Could you check a few things on this model? Use its own coordinates, in mm. A direction names the side the tool comes from. Round coordinates to 2 decimals unless told otherwise and drop trailing zeros. Loops run counter-clockwise (first coordinate to the right, second up) from the corner with the lowest first, then second, coordinate; pieces in that order, holes last. Notation, with made-up numbers: (82, 0.25) - (88, 0.25) arc R31 cw to (88, 39.25) - close; hole circle Ø4 at (89.25, 26). An arc over 180 degrees is marked (long way). Use one line per item in the form item = value.
```python
from build123d import *

# Parameters (mm, degrees)
F0_R          = 1.75
F1_DEPTH      = 1.65
F2_R          = 1
F3_W          = 15.5
F3_H          = 2.5
F4_DEPTH      = 2.25
F5_W          = 0.7
F5_H          = 0.7
F6_DEPTH      = 6
F6_DEPTH_BACK = 6
F7_R          = 0.75


with BuildPart() as f1:
    # F0 (on Top) → F1 (new body)
    with BuildSketch(Plane.XY):
        with BuildLine():
            Line((14.55, 6.8), (-14.55, 6.8))
            Line((-14.55, 6.8), (-14.55, 3.75))
            Line((-14.55, 3.75), (-14.55, 1.8708286934))
            ThreePointArc((-14.55, 1.8708286934), (-14.1771558135, 0.9682458366), (-14.05, 0))
            ThreePointArc((-14.05, 0), (-14.1771558135, -0.9682458366), (-14.55, -1.8708286934))
            Line((-14.55, -1.8708286934), (-14.55, -3.75))
            Line((-14.55, -3.75), (-14.55, -6.8))
            Line((-14.55, -6.8), (14.55, -6.8))
            Line((14.55, -6.8), (14.55, -3.75))
            Line((14.55, -3.75), (14.55, -1.8708286934))
            ThreePointArc((14.55, -1.8708286934), (14.05, 0), (14.55, 1.8708286934))
            Line((14.55, 1.8708286934), (14.55, 3.75))
            Line((14.55, 3.75), (14.55, 6.8))
        make_face()
        with BuildLine():
            Line((-14.55, 1.8708286934), (-14.55, 3.75))
            Line((-14.55, 3.75), (-17.8, 3.75))
            ThreePointArc((-17.8, 3.75), (-15.9229155054, 3.2463908884), (-14.55, 1.8708286934))
        make_face()
        with BuildLine():
            Line((17.8, 3.75), (14.55, 3.75))
            Line((14.55, 3.75), (14.55, 1.8708286934))
            ThreePointArc((14.55, 1.8708286934), (15.9229155054, 3.2463908884), (17.8, 3.75))
        make_face()
        with BuildLine():
            Line((-14.55, -1.8708286934), (-14.55, 1.8708286934))
            ThreePointArc((-14.55, 1.8708286934), (-15.9229155054, 3.2463908884), (-17.8, 3.75))
            ThreePointArc((-17.8, 3.75), (-21.55, 0), (-17.8, -3.75))
            ThreePointArc((-17.8, -3.75), (-15.9229155054, -3.2463908884), (-14.55, -1.8708286934))
        make_face()
        with Locations((-17.8, 0)):
            Circle(F0_R, mode=Mode.SUBTRACT)
        with BuildLine():
            ThreePointArc((17.8, 3.75), (15.9229155054, 3.2463908884), (14.55, 1.8708286934))
            Line((14.55, 1.8708286934), (14.55, -1.8708286934))
            ThreePointArc((14.55, -1.8708286934), (15.9229155054, -3.2463908884), (17.8, -3.75))
            ThreePointArc((17.8, -3.75), (20.4516504294, -2.6516504294), (21.55, 0))
            ThreePointArc((21.55, 0), (20.4516504294, 2.6516504294), (17.8, 3.75))
        make_face()
        with Locations((17.8, 0)):
            Circle(F0_R, mode=Mode.SUBTRACT)
        with BuildLine():
            Line((-14.55, -3.75), (-14.55, -1.8708286934))
            ThreePointArc((-14.55, -1.8708286934), (-15.9229155054, -3.2463908884), (-17.8, -3.75))
            Line((-17.8, -3.75), (-14.55, -3.75))
        make_face()
        with BuildLine():
            ThreePointArc((17.8, -3.75), (15.9229155054, -3.2463908884), (14.55, -1.8708286934))
            Line((14.55, -1.8708286934), (14.55, -3.75))
            Line((14.55, -3.75), (17.8, -3.75))
        make_face()
        with BuildLine():
            ThreePointArc((-14.05, 0), (-14.1771558135, 0.9682458366), (-14.55, 1.8708286934))
            Line((-14.55, 1.8708286934), (-14.55, -1.8708286934))
            ThreePointArc((-14.55, -1.8708286934), (-14.1771558135, -0.9682458366), (-14.05, 0))
        make_face()
        with BuildLine():
            Line((14.55, -1.8708286934), (14.55, 1.8708286934))
            ThreePointArc((14.55, 1.8708286934), (14.05, 0), (14.55, -1.8708286934))
        make_face()
    extrude(amount=F1_DEPTH)

    # F2
    f2_edges = [f1.edges().sort_by_distance(p)[0] for p in [
        (14.55, 3.75, 0.825),
        (14.55, -3.75, 0.825),
        (-14.55, -3.75, 0.825),
        (-14.55, 3.75, 0.825),
    ]]
    fillet(f2_edges, radius=F2_R)

    # F3 (on face) → F4 (join)
    with BuildSketch(Plane(origin=(0, 0, 0), x_dir=(1, 0, 0), z_dir=(0, 0, -1))):
        with Locations((0, 5.55)):
            Rectangle(F3_W, F3_H)
    extrude(amount=F4_DEPTH)

    # F5 (on face) → F6 (join, two sides)
    with BuildSketch(Plane(origin=(0, 0, -2.25), x_dir=(1, 0, 0), z_dir=(0, 0, -1))) as f6_sk:
        with Locations((-6.4, 5.55)):
            Rectangle(F5_W, F5_H)
        with Locations((6.4, 5.55)):
            Rectangle(F5_W, F5_H)
        with Locations((-3.84, 5.55)):
            Rectangle(F5_W, F5_H)
        with Locations((-1.28, 5.55)):
            Rectangle(F5_W, F5_H)
        with Locations((1.28, 5.55)):
            Rectangle(F5_W, F5_H)
        with Locations((3.84, 5.55)):
            Rectangle(F5_W, F5_H)
    extrude(amount=F6_DEPTH)
    extrude(f6_sk.sketch, amount=-F6_DEPTH_BACK)

    # F7
    f7_edges = [f1.edges().sort_by_distance(p)[0] for p in [
        (6.4, -5.2, 1.65),
        (6.75, -5.55, 1.65),
        (6.4, -5.9, 1.65),
        (6.05, -5.55, 1.65),
        (4.19, -5.55, 1.65),
        (3.84, -5.9, 1.65),
        (3.49, -5.55, 1.65),
        (3.84, -5.2, 1.65),
        (1.28, -5.2, 1.65),
        (0.93, -5.55, 1.65),
        (1.28, -5.9, 1.65),
        (1.63, -5.55, 1.65),
        (-1.28, -5.9, 1.65),
        (-1.63, -5.55, 1.65),
        (-0.93, -5.55, 1.65),
        (-1.28, -5.2, 1.65),
        (-3.84, -5.9, 1.65),
        (-4.19, -5.55, 1.65),
        (-3.49, -5.55, 1.65),
        (-3.84, -5.2, 1.65),
        (-6.4, -5.2, 1.65),
        (-6.75, -5.55, 1.65),
        (-6.4, -5.9, 1.65),
        (-6.05, -5.55, 1.65),
    ]]
    fillet(f7_edges, radius=F7_R)


solid = f1.part
```
1. Please list where these lines run through material, in increasing order: line 1 along Y through (x, z) = (17.8, 1.35); line 2 along Z through (x, y) = (4, 0).
Solution:
line_1 = -3.75 to -1.75, 1.75 to 3.75
line_2 = 0 to 1.65
2. If we section it at A-A, the plane z = -6: Write out the boundary of the cut face in (x, y).
Solution:
outline = (-6.75, -5.9) - (-6.05, -5.9) - (-6.05, -5.2) - (-6.75, -5.2) - close; (-4.19, -5.9) - (-3.49, -5.9) - (-3.49, -5.2) - (-4.19, -5.2) - close; (-1.63, -5.9) - (-0.93, -5.9) - (-0.93, -5.2) - (-1.63, -5.2) - close; (0.93, -5.9) - (1.63, -5.9) - (1.63, -5.2) - (0.93, -5.2) - close; (3.49, -5.9) - (4.19, -5.9) - (4.19, -5.2) - (3.49, -5.2) - close; (6.05, -5.9) - (6.75, -5.9) - (6.75, -5.2) - (6.05, -5.2) - close
3. On a 3-axis mill with a long thin cutter (end or side, diameter ignored), from which of +Z, -Z, +X, -X, +Y, -Y can I reach the whole of each face in a straight line? I mean faces 4 (the face through (-17, 3.75, 1)), 5 (the face through (-17, -3.75, 1)), 6 (the face through (14.55, -6, 1)), 7 (the face through (0, -4.3, -1)). Say none if no direction works.
Solution:
face_4 = +Z, -Z, -X, +Y
face_5 = +Z, -Z, -X, -Y
face_6 = +Z, -Z, +X, -Y
face_7 = -Z, +X, -X, +Y
4. If we section it at D-D, the plane y = 4.25: Write out the boundary of the cut face in (x, z), plus the area to 3 significant figures.
Solution:
outline = (-14.68, 0) - (14.68, 0) - (14.68, 1.65) - (-14.68, 1.65) - close
area = 48.5 mm^2
5. For P1, Ø0.8, axis at x = -1, z = 3, coming from the +Y side; P2, Ø0.6, axis at y = -5.5, z = -5, coming from the +X side; P3, Ø0.8, axis at x = 1, z = 3, coming from the -Y side; P4, Ø7, axis at x = -6.5, y = -3.5, coming from the -Z side, each with a flat end and sliding along its axis, tell me the tip position at first contact or that it passes through.
Solution:
P1 = -5.2
P2 = 6.75
P3 = -5.9
P4 = -8.25
6. If we section it at B-B, the plane x = 18.5: Write out the boundary of the cut face in (y, z), plus the area to 3 significant figures.
Solution:
outline = (-3.68, 0) - (-1.6, 0) - (-1.6, 1.65) - (-3.68, 1.65) - close; (1.6, 0) - (3.68, 0) - (3.68, 1.65) - (1.6, 1.65) - close
area = 6.86 mm^2
7. If we section it at C-C, the plane x = 13: Write out the boundary of the cut face in (y, z).
Solution:
outline = (-6.8, 0) - (6.8, 0) - (6.8, 1.65) - (-6.8, 1.65) - close
8. We'd pull the mould along X, two halves only. Please class faces 1 (the face through (0, 6.8, 1)), 2 (the face through (16.41, -1.06, 0.81)), 3 (the face through (-7.75, -6, -1)): +X half, -X half, draft (parallel to the pull), parting line (faces both ways), or undercut.
Solution:
face_1 = draft
face_2 = undercut
face_3 = -X half
